Can you work these out from the model? Positions are in its coordinate system, mm. Round coordinates to 2 decimals unless told otherwise and drop trailing zeros. Write each loop counter-clockwise with the first axis right and the second up, starting at its lowest first coordinate (ties: lowest second). Pieces come first, ordered by that corner, then holes. Notation, with made-up numbers: M 77.25,71 L 82.25,71 A19 cw 82.25,85 Z; hole C 9.25,33.5 d9. An arc over 180 degrees is marked long. Answer as a JSON object with one key per item and string values. Group by question number.
1) I'm going to push flat-ended pins straight in: pin 1 Ø1 at (x, z) = (-12.5, 0.5) entering from +Y; pin 2 Ø1 at (x, z) = (9.5, 1.5) entering from +Y; pin 3 Ø1 at (x, z) = (-4, 1.5) entering from +Y. Where does each tip first touch, or does it pass through?
2) Please list where these lines run through material, in increasing order: L1, parallel to Y at x = 0, z = 1.5; L2, parallel to Y at x = -10, z = 1.45. Write a range as [from, to].
3) If we mould it in two halves opening along Y, with no side actions, what happens to faces 1 (the cylindrical face through (-2.93, 13.18, 1.01)), 2 (the flat face through (9, 10.3, 0)), 3 (the cylindrical face through (-2.343, -17.847, 1.261))? For each: +Y half, -Y half, draft (parallel to the pull), parting line (faces both ways), or undercut.
4) Suppose I cut it at A-A, the plane y = 0. Write out the boundary of the cut face in (x, z), and give its area (3 significant figures).
5) Suppose I cut it at C-C, the plane z = 1.45. Write out the boundary of the cut face in (x, y), and give its area (3 significant figures).
from build123d import *

# Parameters (mm, degrees)
CYLINDER002_R       = 13.5
CYLINDER002_DEPTH   = 2
CYLINDER001_R       = 18
CYLINDER001_DEPTH   = 2
CUT_PLACEMENT_ANGLE = 180
FILLET_R            = 0.5


with BuildPart() as cylinder002:
    # Cylinder002 → Cylinder002 (new body)
    with BuildSketch(Plane.XY):
        Circle(CYLINDER002_R)
    extrude(amount=CYLINDER002_DEPTH)


with BuildPart() as fillet_body:
    # Cylinder001 → Cylinder001 (new body)
    with BuildSketch(Plane.XY):
        Circle(CYLINDER001_R)
    extrude(amount=CYLINDER001_DEPTH)

    # Cut: cut Cylinder002
    add(cylinder002.part, mode=Mode.SUBTRACT)


with BuildPart() as fillet_body_1:
    # Cut placement: moved
    add(fillet_body.part.moved(Location((0, 0, 2))).rotate(Axis((0, 0, 2), (1, 0, 0)), CUT_PLACEMENT_ANGLE))

    # Fillet
    fillet_edges = [fillet_body_1.edges().sort_by_distance(p)[0] for p in [
        (-18, 0, 0),
    ]]
    fillet(fillet_edges, radius=FILLET_R)


solid = fillet_body_1.part
Results:
{
 "1": {"pin 1": "y = 13.42", "pin 2": "y = 15.59", "pin 3": "y = 17.66"},
 "2": {"L1": "[-18, -13.5], [13.5, 18]", "L2": "[-14.97, -9.07], [9.07, 14.97]"},
 "3": {"face 1": "undercut", "face 2": "draft", "face 3": "parting line"},
 "4": {"outline": "M -18,0.5 A0.5 ccw -17.5,0 L -13.5,0 L -13.5,2 L -18,2 Z; M 13.5,0 L 17.5,0 A0.5 ccw 18,0.5 L 18,2 L 13.5,2 Z", "area": "17.9 mm^2"},
 "5": {"outline": "C 0,0 d36; hole C 0,0 d27", "area": "445 mm^2"}
}
